For this review, take the finished solid that the model builds, in its own axes (mm). Face numbers are marked on the shaded views. Round coordinates to 2 decimals unless told otherwise and drop trailing zeros. Write each loop counter-clockwise with the first axis right and the second up, starting at its lowest first coordinate (ties: lowest second). Pieces come first, ordered by that corner, then holes. Notation, with made-up numbers: M 29,-16 L 45,-16 A13 cw 45,-2 Z; hole C 45.5,19 d7. An arc over 180 degrees is marked long. Answer in a Markdown table with one row per item.
```python
from build123d import *

# Parameters (mm, degrees)
SKETCH2_R                  = 6
BOSS_EXTRUDE1_DEPTH        = 38
M24X2_0_TAPPED_HOLE1_D     = 22
M24X2_0_TAPPED_HOLE1_DEPTH = 38
M24X2_0_TAPPED_HOLE1_TIP   = 6.609466809


with BuildPart() as part:
    # Sketch2 → Boss-Extrude1 (new body)
    with BuildSketch(Plane(origin=(0, 0, 0), x_dir=(1, 0, 0), z_dir=(0, 1, 0))):
        with BuildLine():
            Line((-35, 19), (35, 19))
            ThreePointArc((35, 19), (54, 0), (35, -19))
            Line((35, -19), (-35, -19))
            ThreePointArc((-35, -19), (-54, 0), (-35, 19))
        make_face()
        with Locations(Location((-35, 0, 0), (0, 0, 270))):
            Circle(SKETCH2_R, mode=Mode.SUBTRACT)
        with Locations(Location((35, 0, 0), (0, 0, 90))):
            Circle(SKETCH2_R, mode=Mode.SUBTRACT)
    extrude(amount=BOSS_EXTRUDE1_DEPTH)

    # M24x2.0 Tapped Hole1
    with Locations(Plane.XY.offset(19)):
        with Locations((0, 19)):
            Hole(M24X2_0_TAPPED_HOLE1_D / 2, depth=M24X2_0_TAPPED_HOLE1_DEPTH)
            with Locations((0, 0, -(M24X2_0_TAPPED_HOLE1_DEPTH + M24X2_0_TAPPED_HOLE1_TIP / 2))):  # 118° drill point
                Cone(0, M24X2_0_TAPPED_HOLE1_D / 2, M24X2_0_TAPPED_HOLE1_TIP, mode=Mode.SUBTRACT)


solid = part.part
```
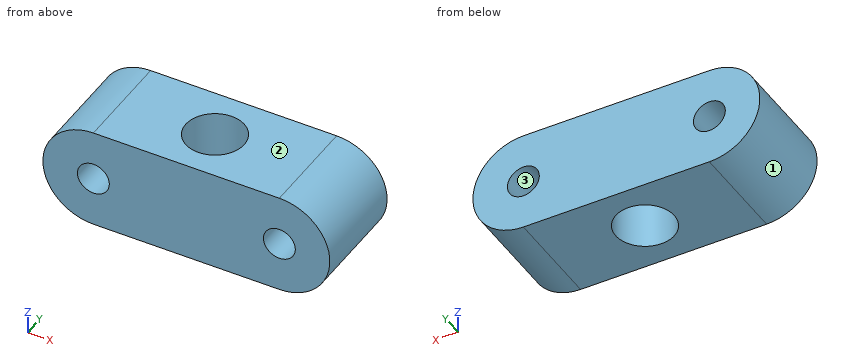
Q1. Take a section at C-C (x = 0). State the section outline as (y, z) points, then the cut area to 3 significant figures.
Found:
| item | result |
|---|---|
| outline | M 0,-19 L 8,-19 L 8,19 L 0,19 Z; M 30,-19 L 38,-19 L 38,19 L 30,19 Z |
| area | 608 mm² |
Q2. Take a section at A-A (y = 19). State the section outline as (x, z) points, then the cut area to 3 significant figures.
Found:
| item | result |
|---|---|
| outline | M -35,-19 L -11,-19 L -11,19 L -35,19 A19 ccw Z; M 11,-19 L 35,-19 A19 ccw 35,19 L 11,19 Z; hole C -35,0 d12; hole C 35,0 d12 |
| area | 2,730 mm² |
Q3. Take a section at B-B (z = 0). State the section outline as (x, y) points.
Found:
| item | result |
|---|---|
| outline | M -54,0 L -41,0 L -41,38 L -54,38 Z; M -29,0 L 29,0 L 29,38 L -29,38 Z; M 41,0 L 54,0 L 54,38 L 41,38 Z; hole C 0,19 d22 |
Q4. Mouldability with a two-part tool opening along X and no side actions: class the marked faces 1, 2 and 3 as +X half, -X half, draft (parallel to the pull), parting line (faces both ways), or undercut.
Found:
| item | result |
|---|---|
| face 1 | -X half |
| face 2 | draft |
| face 3 | undercut |
Q5. Take a section at D-D (y = 5). State the section outline as (x, z) points.
Found:
| item | result |
|---|---|
| outline | M -35,-19 L 35,-19 A19 ccw 35,19 L -35,19 A19 ccw Z; hole C -35,0 d12; hole C 35,0 d12 |
Q6. For probe 1 along X at (y, z) = (23, 0); probe 2 along X at (y, z) = (26, 0); probe 3 along Z at (x, y) = (-34.5, 30), list the stretches that pass through material, from the lowest coordinate up.
Found:
| item | result |
|---|---|
| probe 1 | -54 to -41, -29 to -10.25, 10.25 to 29, 41 to 54 |
| probe 2 | -54 to -41, -29 to -8.49, 8.49 to 29, 41 to 54 |
| probe 3 | -19 to -5.98, 5.98 to 19 |
Q7. Insertion check: P1, Ø1, axis at y = 29, z = -10.5, coming from the -X side; P2, Ø1, axis at y = 32.5, z = 3, coming from the +X side; P3, Ø13, axis at x = 0, y = 19, coming from the -Z side; P4, Ø1, axis at x = 37.5, y = 27.5, coming from the -Z side. Each pin has a flat end and moves straight along its axis. Give the tip position at first contact, or say it passes through.
Found:
| item | result |
|---|---|
| P1 | x = -51.16 |
| P2 | x = 53.83 |
| P3 | through |
| P4 | z = -18.89 |
